Geometry check sheet. Reference: the model listing, model coordinates, mm. A direction names the side the tool comes from. Round coordinates to 2 decimals unless told otherwise and drop trailing zeros. Order: outer loops, then holes, each group sorted by start corner. A loop starts at its lowest first (then second) coordinate and runs counter-clockwise, first axis right, second up.
(1) Sectioned sample at D-D (x = 40). Record the boundary of the cut face in (y, z), plus the area to 3 significant figures.
(2) Sectioned sample at C-C (x = 16). Record the boundary of the cut face in (y, z).
(3) Set-up check for faces 5 (the face through (37.79, -16.67, 2.46)), 6 (the face through (5, -21.25, -10)): record each of +Z, -Z, +X, -X, +Y, -Y from which the full face is reachable in a straight line by a thin tool's end or side.
(4) Go/stop test with flat-tipped pins: pin 1 (3.5 mm diameter, centred on x = 40, y = 18.7, fed in from +Z); pin 2 (7.5 mm diameter, centred on y = -2.5, z = -9.5, fed in from +X); pin 3 (10 mm diameter, centred on y = -4.5, z = -2.5, fed in from -X); pin 4 (5 mm diameter, centred on x = -10.5, z = -8, fed in from -Y). Record where each tip stops, or that it passes through.
(5) Material ranges on line 1 along Y through (x, z) = (40, 2.7); line 2 along Y through (x, z) = (15.5, 2.4); line 3 along Y through (x, z) = (15.5, -16.5), recorded low to high.
(6) Sectioned sample at B-B (y = -18.7). Record the boundary of the cut face in (x, z).
(7) Sectioned sample at A-A (z = 3). Give the number of separate pieces and of enclosed holes in the cut face, plus the area to 3 significant figures.
(8) Release check for a two-part mould opening along Y. For faces 1 (the face through (-16.64, 16.55, 2.46)), 2 (the face through (28.013, -30.648, 2.535)), 3 (the face through (10, 26.25, -7)), 4 (the face through (14.36, -14.45, 2.46)) record: +Y half, -Y half, draft (parallel to the pull), parting line (faces both ways), or undercut.
from build123d import *

# Parameters (mm, degrees)
F0_W     = 42.5
F0_H     = 42.5
F0_R     = 1.55
F0_R_2   = 11.5
F0_W_2   = 6.05
F0_R_3   = 3
F0_R_4   = 6
F1_DEPTH = 5
F2_DEPTH = 25.4
F3_SIZE2 = 42.5
F3_SIZE  = 25.4
F4_R     = 2.5


with BuildPart() as f1:
    # F0 (on Top) → F1 (new body)
    with BuildSketch(Plane.XY):
        Rectangle(F0_W, F0_H)
        with Locations((-15.5, -15.5)):
            Circle(F0_R, mode=Mode.SUBTRACT)
        with Locations((15.5, -15.5)):
            Circle(F0_R, mode=Mode.SUBTRACT)
        with Locations((-15.5, 15.5)):
            Circle(F0_R, mode=Mode.SUBTRACT)
        Circle(F0_R_2, mode=Mode.SUBTRACT)
        with Locations((15.5, 15.5)):
            Circle(F0_R, mode=Mode.SUBTRACT)
        Polygon((-21.25, 21.25), (21.25, 21.25), (27.3, 21.25), (27.3, 26.25), (-21.25, 26.25), align=None)
        with Locations((24.275, 0)):
            Rectangle(F0_W_2, F0_H)
        Polygon((27.3, -21.25), (21.25, -21.25), (-21.25, -21.25), (-21.25, -26.25), (27.3, -26.25), align=None)
        Polygon((27.3, 26.25), (27.3, 21.25), (27.3, -21.25), (27.3, -26.25), (27.3, -31.4), (52.7, -31.4), (52.7, 31.4), (27.3, 31.4), align=None)
        with Locations((40, -18.7)):
            Circle(F0_R_3, mode=Mode.SUBTRACT)
        with Locations((40, 0)):
            Circle(F0_R_4, mode=Mode.SUBTRACT)
        with Locations((40, 18.7)):
            Circle(F0_R_3, mode=Mode.SUBTRACT)
    extrude(amount=F1_DEPTH)

    # F0 (on Top) → F2 (join)
    with BuildSketch(Plane.XY):
        Polygon((27.3, -21.25), (21.25, -21.25), (-21.25, -21.25), (-21.25, -26.25), (27.3, -26.25), align=None)
        with Locations((24.275, 0)):
            Rectangle(F0_W_2, F0_H)
        Polygon((-21.25, 21.25), (21.25, 21.25), (27.3, 21.25), (27.3, 26.25), (-21.25, 26.25), align=None)
    extrude(amount=-F2_DEPTH)

    # F3
    f3_edges = [f1.edges().sort_by_distance(p)[0] for p in [
        (-21.25, -23.75, -25.4),
        (-21.25, 23.75, -25.4),
    ]]
    f3_side = f1.faces().sort_by_distance((-21.25, 0, 4.393336))[0]
    chamfer(f3_edges, length=F3_SIZE, length2=F3_SIZE2, reference=f3_side)

    # F4
    f4_edges = [f1.edges().sort_by_distance(p)[0] for p in [
        (27.3, 31.4, 2.5),
        (52.7, 31.4, 2.5),
        (27.3, 26.25, 2.5),
        (-21.25, 26.25, 2.5),
        (52.7, -31.4, 2.5),
        (27.3, -31.4, 2.5),
        (27.3, -26.25, 2.5),
        (-21.25, -26.25, 2.5),
    ]]
    fillet(f4_edges, radius=F4_R)


solid = f1.part
Answer below:
1. outline: (-31.4, 0) - (-21.7, 0) - (-21.7, 5) - (-31.4, 5) - close; (-15.7, 0) - (-6, 0) - (-6, 5) - (-15.7, 5) - close; (6, 0) - (15.7, 0) - (15.7, 5) - (6, 5) - close; (21.7, 0) - (31.4, 0) - (31.4, 5) - (21.7, 5) - close
1. area: 194 mm2
2. outline: (-26.25, -22.26) - (-21.25, -22.26) - (-21.25, 0) - (-16.97, 0) - (-16.97, 5) - (-26.25, 5) - close; (-14.03, 0) - (14.03, 0) - (14.03, 5) - (-14.03, 5) - close; (16.97, 0) - (21.25, 0) - (21.25, -22.26) - (26.25, -22.26) - (26.25, 5) - (16.97, 5) - close
3. face 5: +Z, -Z
3. face 6: -Z, -X
4. pin 1: passes through
4. pin 2: stops at x = 27.3
4. pin 3: stops at x = -21.25
4. pin 4: stops at y = -26.25
5. line 1: y = -31.4 to -21.7, -15.7 to -6, 6 to 15.7, 21.7 to 31.4
5. line 2: y = -26.25 to -17.05, -13.95 to 13.95, 17.05 to 26.25
5. line 3: y = -26.25 to -21.25, 21.25 to 26.25
6. outline: (-21.25, 0) - (21.25, 0) - (21.25, -25.4) - (27.3, -25.4) - (27.3, 0) - (37, 0) - (37, 5) - (-21.25, 5) - close; (43, 0) - (52.7, 0) - (52.7, 5) - (43, 5) - close
7. separate pieces: 1
7. enclosed holes: 8
7. area: 3,520 mm2
8. face 1: undercut
8. face 2: -Y half
8. face 3: +Y half
8. face 4: undercut
